Source: CAD feature listing. Evaluate the final solid. Frame: model axes, mm. Round coordinates to 2 decimals unless told otherwise and drop trailing zeros. Write each loop counter-clockwise with the first axis right and the second up, starting at its lowest first coordinate (ties: lowest second). Pieces come first, ordered by that corner, then holes.
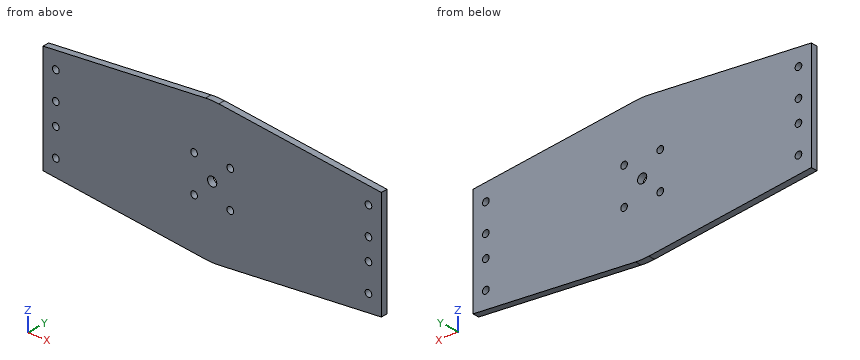
from build123d import *

# Parameters (mm, degrees)
EXTRUDE_1_DEPTH     = 3
SKETCH_2_R          = 1.55
SKETCH_2_R_2        = 2.15
CUT_EXTRUDE_1_DEPTH = 3
SKETCH_3_R          = 1.55
CUT_EXTRUDE_2_DEPTH = 4


with BuildPart() as part:
    # 草图1 → 凸台-拉伸1 (new body)
    with BuildSketch(Plane(origin=(0, 0, 0), x_dir=(1, 0, 0), z_dir=(0, 1, 0))):
        with BuildLine():
            Line((-79, 25), (-79, -25))
            Line((-79, -25), (-3.133353582, -32.34860268))
            ThreePointArc((-3.133353582, -32.34860268), (0, -32.5), (3.133353582, -32.34860268))
            Line((3.133353582, -32.34860268), (79, -25))
            Line((79, -25), (79, 25))
            Line((79, 25), (3.133353582, 32.34860268))
            ThreePointArc((3.133353582, 32.34860268), (0, 32.5), (-3.133353582, 32.34860268))
            Line((-3.133353582, 32.34860268), (-79, 25))
        make_face()
    extrude(amount=EXTRUDE_1_DEPTH)

    # 草图2 → 切除-拉伸1 (cut)
    with BuildSketch(Plane(origin=(0, 3, 0), x_dir=(1, 0, 0), z_dir=(0, 1, 0))):
        with Locations(Location((-8.45, 8.45, 0), (0, 0, 270))):
            Circle(SKETCH_2_R)
        with Locations(Location((8.45, 8.45, 0), (0, 0, 270))):
            Circle(SKETCH_2_R)
        with Locations(Location((8.45, -8.45, 0), (0, 0, 270))):
            Circle(SKETCH_2_R)
        with Locations(Location((-8.45, -8.45, 0), (0, 0, 270))):
            Circle(SKETCH_2_R)
        with Locations(Location((0, 0, 0), (0, 0, 270))):
            Circle(SKETCH_2_R_2)
    extrude(amount=-CUT_EXTRUDE_1_DEPTH, mode=Mode.SUBTRACT)

    # 草图3 → 切除-拉伸2 (cut)
    with BuildSketch(Plane.XZ):
        with Locations(Location((-73, 17.74, 0), (0, 0, 270))):
            Circle(SKETCH_3_R)
        with Locations(Location((-73, 5, 0), (0, 0, 270))):
            Circle(SKETCH_3_R)
        with Locations(Location((-73, -5, 0), (0, 0, 270))):
            Circle(SKETCH_3_R)
        with Locations(Location((-73, -17.74, 0), (0, 0, 270))):
            Circle(SKETCH_3_R)
    cut_extrude_2 = extrude(amount=-CUT_EXTRUDE_2_DEPTH, mode=Mode.SUBTRACT)

    # 镜向1: 切除-拉伸2 across plane
    add(cut_extrude_2.mirror(Plane(origin=(0, 0, 0), x_dir=(0, 0, 1), z_dir=(1, 0, 0))), mode=Mode.SUBTRACT)


solid = part.part
1) Section query D-D on x = -49.5. Return the cut outline in (y, z).
Taken from the geometry:
outline: (0, -27.86) - (3, -27.86) - (3, 27.86) - (0, 27.86) - close
2) Material intervals for line 1 (X direction, y = 1.25, z = -8.45); line 2 (X direction, y = 0.9, z = -5); line 3 (Z direction, x = 73, y = 2.4), sorted ascending.
Taken from the geometry:
line 1: x = -79 to -10, -6.9 to 6.9, 10 to 79
line 2: x = -79 to -74.55, -71.45 to 71.45, 74.55 to 79
line 3: z = -25.58 to -19.29, -16.19 to -6.55, -3.45 to 3.45, 6.55 to 16.19, 19.29 to 25.58
3) Section query B-B on z = 17.74. Return the cut outline in (x, y), then the cut area to 3 significant figures.
Taken from the geometry:
outline: (-79, 0) - (-74.55, 0) - (-74.55, 3) - (-79, 3) - close; (-71.45, 0) - (71.45, 0) - (71.45, 3) - (-71.45, 3) - close; (74.55, 0) - (79, 0) - (79, 3) - (74.55, 3) - close
area: 455 mm2
4) Contact query for flat-ended pins moving along their axis: P1, Ø4, axis at x = -73, z = -5, coming from the -Y side; P2, Ø1.5, axis at x = -54, y = 1.5, coming from the +Z side. Output: stop coordinate, or through.
Taken from the geometry:
P1: stops at y = 0
P2: stops at z = 27.49
5) Section query C-C on y = 2.1. State how many separate pieces and enclosed holes the cut face has, then the cut area to 3 significant figures.
Taken from the geometry:
separate pieces: 1
enclosed holes: 13
area: 9,000 mm2
6) Section query A-A on x = 0. Return the cut outline in (y, z), then the cut area to 3 significant figures.
Taken from the geometry:
outline: (0, -32.5) - (3, -32.5) - (3, -2.15) - (0, -2.15) - close; (0, 2.15) - (3, 2.15) - (3, 32.5) - (0, 32.5) - close
area: 182 mm2
